Can you work these out from the drawing? Everything is in mm from the part's minimum corner. Round coordinates to 2 decimals unless told otherwise and drop trailing zeros. Order: outer loops, then holes, each group sorted by start corner. A loop starts at its lowest first (then second) coordinate and runs counter-clockwise, first axis right, second up. Notation, with made-up numbers: M -22,40.5 L 24,40.5 A25 ccw 24,63.5 Z; hole C 71.25,14.25 d1. An arc over 180 degrees is marked long. Write each question's results on one line, items separated by ' | '. Start each with the question number.
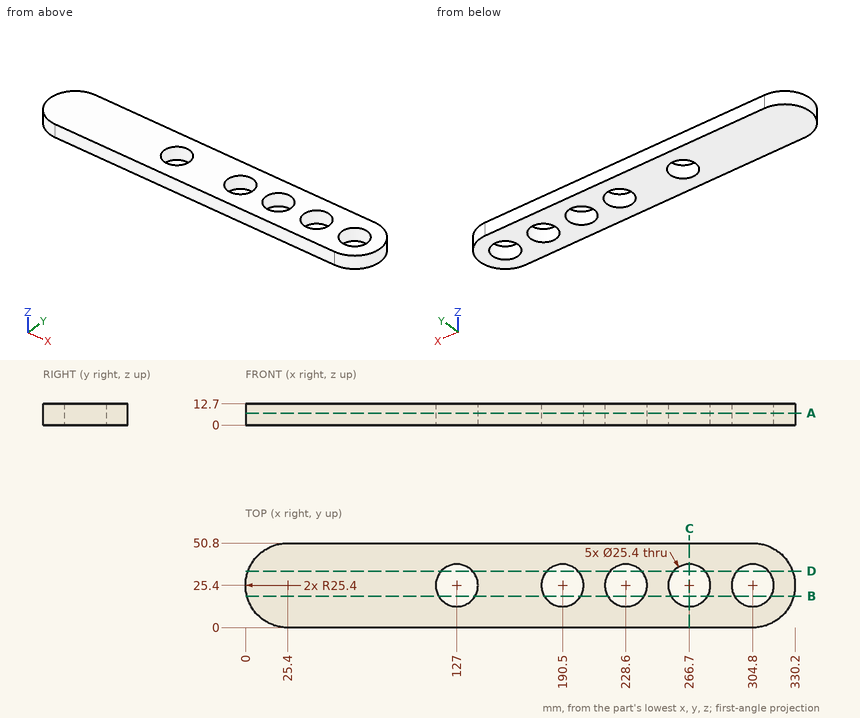
(1) I want a section at A-A on z = 7.25. Write out the boundary of the cut face in (x, y).
(2) I want a section at D-D on y = 34. Write out the boundary of the cut face in (x, z), and give its area (3 significant figures).
(3) I want a section at B-B on y = 19. Write out the boundary of the cut face in (x, z).
(4) I want a section at C-C on x = 266.7. Write out the boundary of the cut face in (y, z).
(5) I'm going to push flat-ended pins straight in: pin 1 Ø15 at (x, y) = (266.7, 25.4) entering from -Z; pin 2 Ø12 at (x, y) = (219, 9.5) entering from -Z; pin 3 Ø4 at (y, z) = (12, 8) entering from +X; pin 4 Ø1 at (y, z) = (11, 6.5) entering from +X. Where does each tip first touch, or does it pass through?
(6) Please list where these lines run through material, in increasing order: line 1 (X direction, y = 25, z = 4.5); line 2 (X direction, y = 16.5, z = 1.75); line 3 (Y direction, x = 266.7, z = 3.75).
Solutions:
1) outline: M 25.4,0 L 304.8,0 A25.4 ccw 304.8,50.8 L 25.4,50.8 A25.4 ccw Z; hole C 127,25.4 d25.4; hole C 190.5,25.4 d25.4; hole C 228.6,25.4 d25.4; hole C 266.7,25.4 d25.4; hole C 304.8,25.4 d25.4
2) outline: M 1.5,0 L 117.65,0 L 117.65,12.7 L 1.5,12.7 Z; M 136.35,0 L 181.15,0 L 181.15,12.7 L 136.35,12.7 Z; M 199.85,0 L 219.25,0 L 219.25,12.7 L 199.85,12.7 Z; M 237.95,0 L 257.35,0 L 257.35,12.7 L 237.95,12.7 Z; M 276.05,0 L 295.45,0 L 295.45,12.7 L 276.05,12.7 Z; M 314.15,0 L 328.7,0 L 328.7,12.7 L 314.15,12.7 Z | area: 2,970 mm^2
3) outline: M 0.82,0 L 116.03,0 L 116.03,12.7 L 0.82,12.7 Z; M 137.97,0 L 179.53,0 L 179.53,12.7 L 137.97,12.7 Z; M 201.47,0 L 217.63,0 L 217.63,12.7 L 201.47,12.7 Z; M 239.57,0 L 255.73,0 L 255.73,12.7 L 239.57,12.7 Z; M 277.67,0 L 293.83,0 L 293.83,12.7 L 277.67,12.7 Z; M 315.77,0 L 329.38,0 L 329.38,12.7 L 315.77,12.7 Z
4) outline: M 0,0 L 12.7,0 L 12.7,12.7 L 0,12.7 Z; M 38.1,0 L 50.8,0 L 50.8,12.7 L 38.1,12.7 Z
5) pin 1: through | pin 2: z = 0 | pin 3: x = 327.5 | pin 4: x = 326.06
6) line 1: 0 to 114.31, 139.69 to 177.81, 203.19 to 215.91, 241.29 to 254.01, 279.39 to 292.11, 317.49 to 330.2 | line 2: 1.61 to 117.94, 136.06 to 181.44, 199.56 to 219.54, 237.66 to 257.64, 275.76 to 295.74, 313.86 to 328.59 | line 3: 0 to 12.7, 38.1 to 50.8
